For this review, take the finished solid that the model builds, in its own axes (mm). A direction names the side the tool comes from. Coordinates: 2 decimals unless noted, no trailing zeros. Loops run counter-clockwise (first coordinate to the right, second up) from the corner with the lowest first, then second, coordinate; pieces in that order, holes last. Notation, with made-up numbers: M 56,44 L 97,44 A20 ccw 97,73 Z; hole C -1,-25.5 d1. An arc over 180 degrees is marked long. Write item = value, one per line.
from build123d import *

# Parameters (mm, degrees)
MODEL_R                         = 1.7
MODEL_R_2                       = 11.05
AUFSATZ_LINEAR_AUSTRAGEN1_DEPTH = 3


with BuildPart() as part:
    # Model → Aufsatz-Linear austragen1 (new body)
    with BuildSketch(Plane.XY):
        with BuildLine():
            Line((51, 3), (51, 23.65151519))
            Line((51, 23.65151519), (56.870057685, 29.521572875))
            ThreePointArc((56.870057685, 29.521572875), (58.04163056, 32.35), (56.870057685, 35.178427125))
            Line((56.870057685, 35.178427125), (32.828427125, 59.220057685))
            ThreePointArc((32.828427125, 59.220057685), (30, 60.39163056), (27.171572875, 59.220057685))
            Line((27.171572875, 59.220057685), (3.129942315, 35.178427125))
            ThreePointArc((3.129942315, 35.178427125), (1.95836944, 32.35), (3.129942315, 29.521572875))
            Line((3.129942315, 29.521572875), (9, 23.65151519))
            Line((9, 23.65151519), (9, 3))
            ThreePointArc((9, 3), (9.878679656, 0.878679656), (12, 0))
            Line((12, 0), (48, 0))
            ThreePointArc((48, 0), (50.121320344, 0.878679656), (51, 3))
        make_face()
        with Locations((30, 10.429689783)):
            Circle(MODEL_R, mode=Mode.SUBTRACT)
        with Locations((51.920310217, 32.35)):
            Circle(MODEL_R, mode=Mode.SUBTRACT)
        with Locations((30, 54.270310217)):
            Circle(MODEL_R, mode=Mode.SUBTRACT)
        with Locations((8.079689783, 32.35)):
            Circle(MODEL_R, mode=Mode.SUBTRACT)
        with Locations((30, 32.35)):
            Circle(MODEL_R_2, mode=Mode.SUBTRACT)
        with BuildLine():
            Line((22.7, 10), (22.7, 17.5))
            ThreePointArc((22.7, 17.5), (20, 20.2), (17.3, 17.5))
            Line((17.3, 17.5), (17.3, 10))
            ThreePointArc((17.3, 10), (20, 7.3), (22.7, 10))
        make_face(mode=Mode.SUBTRACT)
        with BuildLine():
            Line((37.3, 10), (37.3, 17.5))
            ThreePointArc((37.3, 17.5), (40, 20.2), (42.7, 17.5))
            Line((42.7, 17.5), (42.7, 10))
            ThreePointArc((42.7, 10), (40, 7.3), (37.3, 10))
        make_face(mode=Mode.SUBTRACT)
    extrude(amount=AUFSATZ_LINEAR_AUSTRAGEN1_DEPTH)


solid = part.part
Q1. Add section B-B (x = 36.5). Write out the cut boundary in (y, z), and give its area (3 significant figures).
Solved:
outline = M 0,0 L 23.41,0 L 23.41,3 L 0,3 Z; M 41.29,0 L 55.55,0 L 55.55,3 L 41.29,3 Z
area = 113 mm²
Q2. Draft analysis for pull direction X (two halves, no side actions). For faces 1 (the face through (58.04, 32.31, 1.48)), 2 (the face through (42.7, 14, 1)), 3 (the face through (30, 0, 1)), state which applies: +X half, -X half, draft (parallel to the pull), parting line (faces both ways), or undercut.
Solved:
face_1 = +X half
face_2 = undercut
face_3 = draft
Q3. Add section A-A (x = 30). Write out the cut boundary in (y, z), and give its area (3 significant figures).
Solved:
outline = M 0,0 L 8.73,0 L 8.73,3 L 0,3 Z; M 12.13,0 L 21.3,0 L 21.3,3 L 12.13,3 Z; M 43.4,0 L 52.57,0 L 52.57,3 L 43.4,3 Z; M 55.97,0 L 60.39,0 L 60.39,3 L 55.97,3 Z
area = 94.5 mm²
Q4. For line 1 along Y through (x, z) = (30, 2.15); line 2 along X through (y, z) = (14.5, 0.25); line 3 along Y through (x, z) = (30.5, 0.2), list the stretches that pass through material, from the lowest coordinate up.
Solved:
line_1 = 0 to 8.73, 12.13 to 21.3, 43.4 to 52.57, 55.97 to 60.39
line_2 = 9 to 17.3, 22.7 to 37.3, 42.7 to 51
line_3 = 0 to 8.8, 12.05 to 21.31, 43.39 to 52.65, 55.9 to 60.36
Q5. For pin 1 Ø3 at (x, y) = (35.5, 11) entering from -Z; pin 2 Ø1.5 at (y, z) = (21.5, 2.5) entering from -X, all flat-tipped, find the tip position at first contact; note any pin that passes through.
Solved:
pin_1 = 0
pin_2 = 9
Q6. Add section C-C (y = 36.5). Write out the cut boundary in (x, z).
Solved:
outline = M 4.45,0 L 19.76,0 L 19.76,3 L 4.45,3 Z; M 40.24,0 L 55.55,0 L 55.55,3 L 40.24,3 Z
Q7. Add section D-D (z = 2). Write out the cut boundary in (x, y), and give its area (3 significant figures).
Solved:
outline = M 3.13,29.52 L 9,23.65 L 9,3 A3 ccw 12,0 L 48,0 A3 ccw 51,3 L 51,23.65 L 56.87,29.52 A4 ccw 56.87,35.18 L 32.83,59.22 A4 ccw 27.17,59.22 L 3.13,35.18 A4 ccw Z; hole C 8.08,32.35 d3.4; hole M 17.3,10 A2.7 ccw 22.7,10 L 22.7,17.5 A2.7 ccw 17.3,17.5 Z; hole C 30,32.35 d22.1; hole C 30,10.43 d3.4; hole C 30,54.27 d3.4; hole M 37.3,10 A2.7 ccw 42.7,10 L 42.7,17.5 A2.7 ccw 37.3,17.5 Z; hole C 51.92,32.35 d3.4
area = 1,760 mm²
Q8. Machinability: for faces 4 (the face through (30, 17, 0)), 5 (the face through (22.7, 14, 1)), 6 (the face through (51, 13, 1)), which of the approach directions +Z, -Z, +X, -X, +Y, -Y give a long, thin tool a straight path to every point of the face, cutting with its end or side? Answer none if there is none.
Solved:
face_4 = -Z, +X, -X, +Y, -Y
face_5 = +Z, -Z
face_6 = +Z, -Z, +X, -Y
